Autodesk Inventor part; units mm, degrees
ref_plane "YZ Plane" through (0, 0, 0) normal (1, 0, 0) x (0, 1, 0)
ref_plane "XZ Plane" through (0, 0, 0) normal (0, 1, 0) x (-1, 0, 0)
ref_plane "XY Plane" through (0, 0, 0) normal (0, 0, 1) x (1, 0, 0)
sketch "スケッチ1" plane through (0, 0, 0) normal (0, 0, 1) x (1, 0, 0)
  circle A0 centre (0, 0) radius 22
  dimension "d0" = 44
extrude "プレート1" add sketch "スケッチ1" along normal mid plane 3.2
sketch "スケッチ2" plane through (0, 0, 1.6) normal (0, 0, 1) x (1, 0, 0)
  line L0 (-10, -10) -> (10, -10)
  line L1 (10, -10) -> (10, 10)
  line L2 (10, 10) -> (-10, 10)
  line L3 (-10, 10) -> (-10, -10)
  line L4 (-10, -10) -> (10, 10) construction
  line L5 (10, -10) -> (-10, 10) construction
  point P0 (0, 0)
  dimension "d2" = 20
  dimension "d3" = 20
hole "穴1" at (-10, 10, 1.6) at (10, 10, 1.6) at (10, -10, 1.6) at (-10, -10, 1.6) direction (0, 0, -1) diameter 5.5 depth 3.2 tip angle 118
equation "\"d9\" = Thickness"
equation "\"d1\" = Thickness"
equation "\"BendRadius\" = Thickness"
equation "\"BendReliefWidth\" = Thickness"
equation "\"BendReliefDepth\" = 0.5 * Thickness"
equation "\"CornerReliefSize\" = 4 * Thickness"
equation "\"MinimumRemnant\" = 2 * Thickness"
equation "\"TransitionRadius\" = BendRadius"
equation "\"JacobiRadiusSize\" = BendRadius"
equation "\"GapSize\" = Thickness"
properties part number "scara-plate2" material "鋼、炭素鋼"
Verification items for the finished model (mm, model axes). Coordinates: 2 decimals unless noted, no trailing zeros. Order: outer loops, then holes, each group sorted by start corner. A loop starts at its lowest first (then second) coordinate and runs counter-clockwise, first axis right, second up.
Item 1: Section check D-D, the plane x = 16. Enter the section's corners in (y, z), then the cut area to 3 significant figures.
Filled in:
outline: (-15.1, -1.6) - (15.1, -1.6) - (15.1, 1.6) - (-15.1, 1.6) - close
area: 96.6 mm2
Item 2: Section check B-B, the plane x = -8. Enter the section's corners in (y, z).
Filled in:
outline: (-20.49, -1.6) - (-11.89, -1.6) - (-11.89, 1.6) - (-20.49, 1.6) - close; (-8.11, -1.6) - (8.11, -1.6) - (8.11, 1.6) - (-8.11, 1.6) - close; (11.89, -1.6) - (20.49, -1.6) - (20.49, 1.6) - (11.89, 1.6) - close
Item 3: Material ranges on L1, parallel to X at y = -10, z = 0.3; L2, parallel to X at y = 7.5, z = 0, recorded low to high.
Filled in:
L1: x = -19.6 to -12.75, -7.25 to 7.25, 12.75 to 19.6
L2: x = -20.68 to -11.15, -8.85 to 8.85, 11.15 to 20.68
Item 4: Section check A-A, the plane y = -11.5. Enter the section's corners in (x, z) (3 decimals).
Filled in:
outline: (-18.755, -1.6) - (-12.305, -1.6) - (-12.305, 1.6) - (-18.755, 1.6) - close; (-7.695, -1.6) - (7.695, -1.6) - (7.695, 1.6) - (-7.695, 1.6) - close; (12.305, -1.6) - (18.755, -1.6) - (18.755, 1.6) - (12.305, 1.6) - close
Item 5: Section check C-C, the plane z = 0.25. Enter the section's corners in (x, y).
Filled in:
outline: circle Ø44 at (0, 0); hole circle Ø5.5 at (-10, -10); hole circle Ø5.5 at (-10, 10); hole circle Ø5.5 at (10, -10); hole circle Ø5.5 at (10, 10)
Item 6: Depth check by flat-ended pin: pin 1 (3 mm diameter, centred on x = -10.5, y = -10.5, fed in from -Z). Enter the tip coordinate at first touch or a pass-through.
Filled in:
pin 1: passes through
Item 7: Release check for a two-part mould opening along Y. For faces 1 (the face through (-12.32, -11.48, -0.02)), 2 (the face through (-4.769, -21.477, 0.022)), 3 (the face through (0, 0, 1.6)), 4 (the face through (11.05, 7.46, -0.02)) record: +Y half, -Y half, draft (parallel to the pull), parting line (faces both ways), or undercut.
Filled in:
face 1: undercut
face 2: parting line
face 3: draft
face 4: undercut
